Can you work these out from the model? Positions are in its coordinate system, mm. Round coordinates to 2 decimals unless told otherwise and drop trailing zeros. Order: outer loops, then holes, each group sorted by start corner. A loop starts at its lowest first (then second) coordinate and runs counter-clockwise, first axis right, second up. Notation, with made-up numbers: (24, 3) -> (37, 3) arc R7 cw to (37, 15) -> close; hole circle Ø4 at (-16, -30.75). An arc over 180 degrees is marked (long way). One line per item, written item: value.
```python
from build123d import *

# Parameters (mm, degrees)
SKETCH_2_W          = 180.073706553
SKETCH_2_H          = 255.410665416
EXTRUDE_1_DEPTH     = 3
CUT_EXTRUDE_1_DEPTH = 3
SKETCH_5_W          = 5
SKETCH_5_H          = 51.907374001
CUT_EXTRUDE_2_DEPTH = 3
MM_TRANSITIONAL_1_D = 3
MM_TRANSITIONAL_2_D = 3
MM_1_D              = 3
MM_2_D              = 3
MM_3_D              = 3


with BuildPart() as part:
    # 草图2 → 凸台-拉伸1 (new body)
    with BuildSketch(Plane(origin=(0, 0, 0), x_dir=(1, 0, 0), z_dir=(0, 1, 0))):
        with Locations((-186.026538889, 60.786498031)):
            Rectangle(SKETCH_2_W, SKETCH_2_H)
    extrude(amount=EXTRUDE_1_DEPTH)

    # 草图4 → 切除-拉伸1 (cut)
    with BuildSketch(Plane(origin=(0, 3, 0), x_dir=(1, 0, 0), z_dir=(0, 1, 0))):
        Polygon((-276.063392165, 188.491830739), (-276.063392165, 169.449737011), (-257.021298437, 188.491830739), align=None)
        Polygon((-182.318869317, 174.967222445), (-115.03177934, 188.491830739), (-257.021298437, 188.491830739), align=None)
        Polygon((-95.989685612, -66.918834677), (-95.989685612, -47.876740949), (-115.03177934, -66.918834677), align=None)
        Polygon((-101.507171046, 174.967222445), (-95.989685612, 169.449737011), (-95.989685612, 188.491830739), (-115.03177934, 188.491830739), align=None)
        Polygon((-276.063392165, -66.918834677), (-257.021298437, -66.918834677), (-276.063392165, -47.876740949), align=None)
    extrude(amount=-CUT_EXTRUDE_1_DEPTH, mode=Mode.SUBTRACT)

    # 草图5 → 切除-拉伸2 (cut)
    with BuildSketch(Plane(origin=(0, 3, 0), x_dir=(1, 0, 0), z_dir=(0, 1, 0))):
        with Locations((-273.563392165, -21.923053949)):
            Rectangle(SKETCH_5_W, SKETCH_5_H)
        with Locations((-98.489685612, -21.923053949)):
            Rectangle(SKETCH_5_W, SKETCH_5_H)
    extrude(amount=-CUT_EXTRUDE_2_DEPTH, mode=Mode.SUBTRACT)

    # 大小mm Transitional 暗销孔1 (through all)
    with Locations(Plane(origin=(0, 3, 0), x_dir=(1, 0, 0), z_dir=(0, 1, 0))):
        with Locations((-254.190617934, 168.879326308), (-254.190617934, 140.929201846), (-225.670082768, 168.879326308), (-225.670082768, 140.929201846), (-150.946280635, 168.879326308), (-150.946280635, 140.929201846)):
            Hole(MM_TRANSITIONAL_1_D / 2)

    # 大小mm Transitional 暗销孔2 (through all)
    with Locations(Plane(origin=(0, 3, 0), x_dir=(1, 0, 0), z_dir=(0, 1, 0))):
        with Locations((-122.425745469, 168.879326308), (-122.425745469, 140.929201846), (-254.190617934, -19.080554812), (-254.190617934, -48.623265957), (-227.646698458, -19.080554812), (-227.646698458, -48.623265957), (-141.859210323, -19.080554812), (-141.859210323, -48.623265957), (-112.884628238, -19.080554812), (-112.884628238, -48.623265957)):
            Hole(MM_TRANSITIONAL_2_D / 2)

    # 大小mm 暗销孔1 (through all)
    with Locations(Plane(origin=(0, 3, 0), x_dir=(1, 0, 0), z_dir=(0, 1, 0))):
        with Locations((-261.411752565, 111.183890873), (-261.411752565, 41.379238152), (-213.780342473, 41.379238152), (-213.780342473, 111.183890873)):
            Hole(MM_1_D / 2)

    # 大小mm 暗销孔2 (through all)
    with Locations(Plane(origin=(0, 0, 0), x_dir=(-1, 0, 0), z_dir=(0, -1, 0))):
        with Locations((202.317574636, -49.390676976), (169.34910988, -49.390676976), (183.870933642, -28.589145642)):
            Hole(MM_2_D / 2)

    # 大小mm 暗销孔3 (through all)
    with Locations(Plane(origin=(0, 0, 0), x_dir=(-1, 0, 0), z_dir=(0, -1, 0))):
        with Locations((199.707102637, 148.354982104), (187.707102637, 148.354982104), (199.707102637, 160.354982104), (187.707102637, 160.354982104)):
            Hole(MM_3_D / 2)


solid = part.part
```
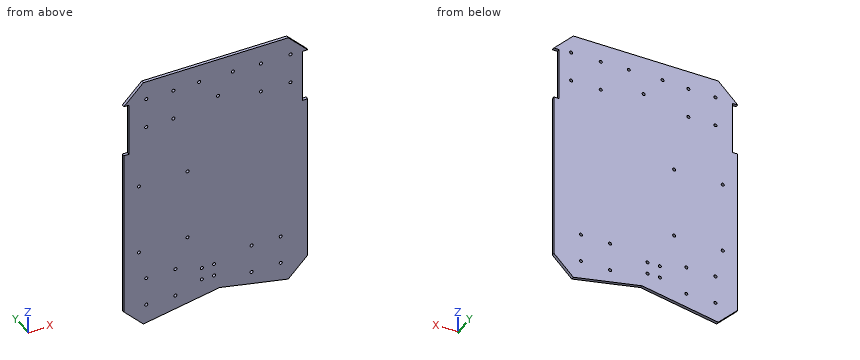
Q1. I want a section at A-A on z = 40.5. List the corners of the cut face in (x, y) for me, plus the area to 3 significant figures.
Answers below:
outline: (-271.06, 0) -> (-100.99, 0) -> (-100.99, 3) -> (-271.06, 3) -> close
area: 510 mm^2
Q2. I want a section at C-C on x = -134.5. List the corners of the cut face in (y, z) for me.
Answers below:
outline: (0, -184.58) -> (3, -184.58) -> (3, 66.92) -> (0, 66.92) -> close
Q3. I want a section at B-B on y = 0.6. Give the number of separate pieces and of enclosed holes in the cut face, plus the area to 3 significant figures.
Answers below:
separate pieces: 1
enclosed holes: 27
area: 43,600 mm^2
Q4. Will these pins go through, and if not, where does the flat tip stop? pin 1 Ø2.5 at (x, z) = (-254.19, -168.88) entering from +Y (3 decimals); pin 2 Ø1.5 at (y, z) = (2, 29.5) entering from -X; pin 3 Ø1.5 at (y, z) = (1.5, 15.5) entering from +X.
Answers below:
pin 1: through
pin 2: x = -271.06
pin 3: x = -100.99
Q5. Please list where these lines run through material, in increasing order: line 1 along Z through (x, y) = (-254.5, 2); line 2 along Z through (x, y) = (-141.5, 2.65); line 3 along Z through (x, y) = (-253.5, 2.15).
Answers below:
line 1: -188.04 to -170.35, -167.41 to -142.4, -139.46 to 17.61, 20.55 to 47.16, 50.09 to 66.92
line 2: -183.17 to 17.62, 20.54 to 47.17, 50.08 to 66.92
line 3: -187.85 to -170.21, -167.55 to -142.26, -139.6 to 17.75, 20.41 to 47.29, 49.95 to 66.92
